Answer from the drawing. Dimensions are ordinates in mm from the lowest x, y and z of the part. A direction names the side the tool comes from. Give positions to 0.01 mm unless a question says otherwise; leave off trailing zeros. Order: outer loops, then holes, each group sorted by start corner. A loop starts at its lowest first (then second) coordinate and runs counter-clockwise, first axis right, second up. Notation, with made-up numbers: (8, 68.5) -> (25, 68.5) arc R4 cw to (25, 74.5) -> close; hole circle Ø3 at (65, -13.5). An arc over 180 degrees is marked (long way). One line per question, with ' | ' between items. Start each with the question number.
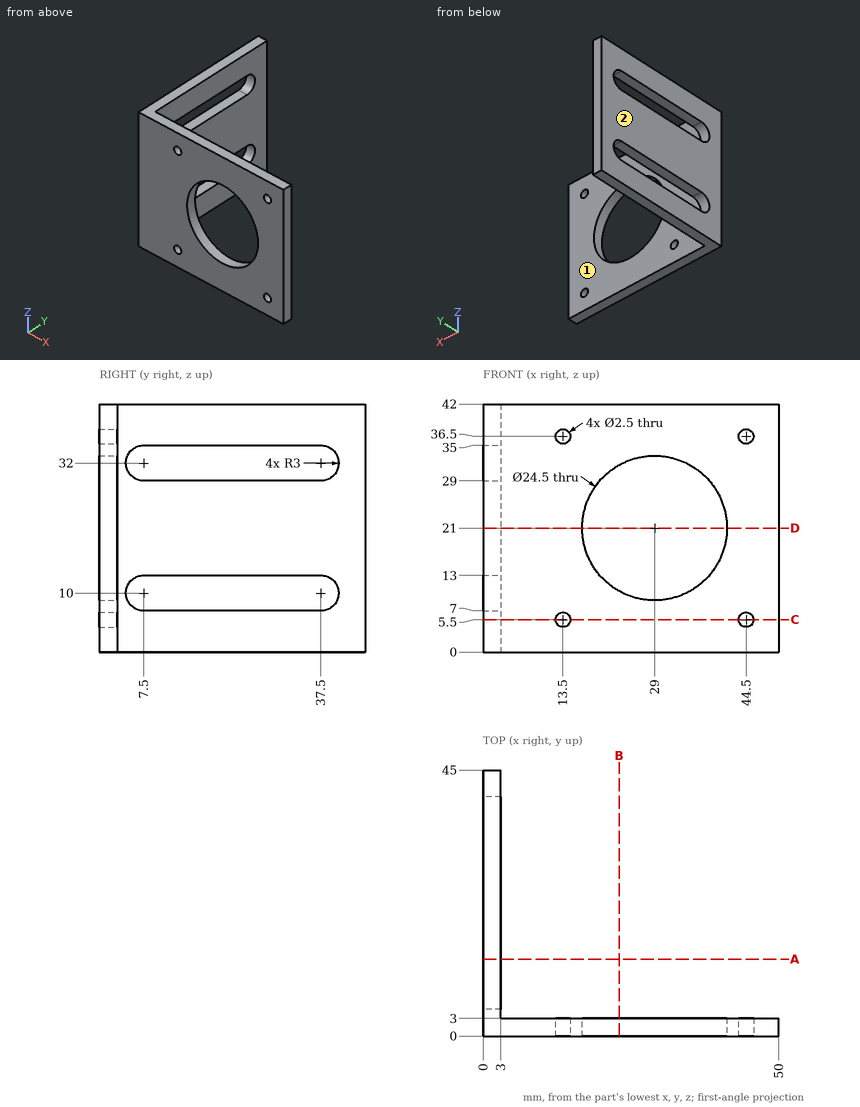
(1) Given P1, Ø1.5, axis at x = 1.5, y = 17, coming from the -Z side; P2, Ø3, axis at x = 44.5, z = 5.5, coming from the +Y side, each flat-ended and moving along its own axis, determine where each tip first touches the part or whether it passes through.
(2) The part is cut by section D-D on z = 21. Determine the outline of the cut face in (x, y).
(3) The part is cut by section A-A on y = 13. Determine the outline of the cut face in (x, z), plus the area to 3 significant figures.
(4) The part is cut by section C-C on z = 5.5. Determine the outline of the cut face in (x, y).
(5) The part is cut by section B-B on x = 23. Determine the outline of the cut face in (y, z), plus the area to 3 significant figures.
(6) For the marked faces 1 and 2, determine the directions among +Z, -Z, +X, -X, +Y, -Y from which every point of the face is accessible in a straight line to the end or side of a thin tool.
(7) Consider line 1 (Z direction, x = 44.5, y = 1.65); line 2 (Z direction, x = 13, y = 1); line 3 (X direction, y = 26, z = 16.5). Determine where each line is inside the solid, lowest interval first.
Result sheet:
1) P1: stops at z = 0 | P2: stops at y = 3
2) outline: (0, 0) -> (16.75, 0) -> (16.75, 3) -> (3, 3) -> (3, 45) -> (0, 45) -> close; (41.25, 0) -> (50, 0) -> (50, 3) -> (41.25, 3) -> close
3) outline: (0, 0) -> (3, 0) -> (3, 7) -> (0, 7) -> close; (0, 13) -> (3, 13) -> (3, 29) -> (0, 29) -> close; (0, 35) -> (3, 35) -> (3, 42) -> (0, 42) -> close | area: 90.0 mm^2
4) outline: (0, 0) -> (12.25, 0) -> (12.25, 3) -> (3, 3) -> (3, 45) -> (0, 45) -> close; (14.75, 0) -> (43.25, 0) -> (43.25, 3) -> (14.75, 3) -> close; (45.75, 0) -> (50, 0) -> (50, 3) -> (45.75, 3) -> close
5) outline: (0, 0) -> (3, 0) -> (3, 10.32) -> (0, 10.32) -> close; (0, 31.68) -> (3, 31.68) -> (3, 42) -> (0, 42) -> close | area: 61.9 mm^2
6) face 1: +Z, -Z, +X, +Y | face 2: +Z, -Z, -X, +Y, -Y
7) line 1: z = 0 to 4.25, 6.75 to 35.25, 37.75 to 42 | line 2: z = 0 to 4.35, 6.65 to 35.35, 37.65 to 42 | line 3: x = 0 to 3
